Design review of the part built by this model. Coordinates are the model's own, in mm. Face numbers are marked on the shaded views. A direction names the side the tool comes from. Coordinates: 2 decimals unless noted, no trailing zeros. Loops run counter-clockwise (first coordinate to the right, second up) from the corner with the lowest first, then second, coordinate; pieces in that order, holes last. Notation, with made-up numbers: (-13.75, 22) -> (33.25, 22) arc R26 cw to (33.25, 36) -> close; hole circle Ø8 at (7.25, 0.5). An arc over 180 degrees is marked (long way). Answer as a JSON object with one key per item and string values.
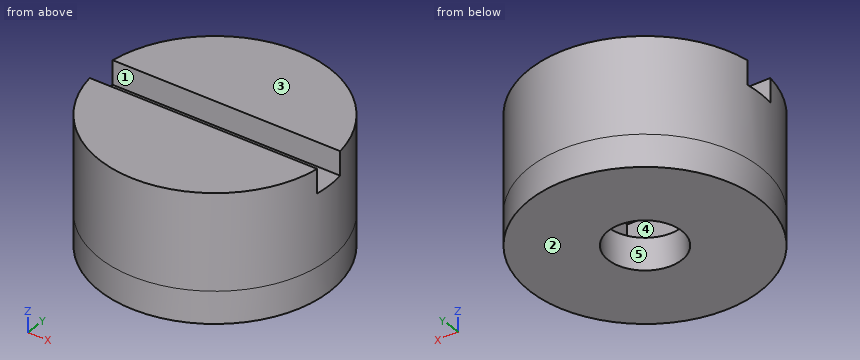
```python
from build123d import *

# Parameters (mm, degrees)
SKETCH_R        = 7.2
SKETCH_R_2      = 2.3
PAD_DEPTH       = 2
SKETCH001_R     = 7.2
PAD001_DEPTH    = 6
SKETCH002_W     = 8
SKETCH002_H     = 8
POCKET_DEPTH    = 3
SKETCH003_W     = 26.953154
SKETCH003_H     = 2
POCKET001_DEPTH = 3.5


with BuildPart() as part:
    # Sketch → Pad (new body)
    with BuildSketch(Plane.XY):
        Circle(SKETCH_R)
        Circle(SKETCH_R_2, mode=Mode.SUBTRACT)
    extrude(amount=-PAD_DEPTH)

    # Sketch001 → Pad001 (join)
    with BuildSketch(Plane.XY):
        Circle(SKETCH001_R)
    extrude(amount=PAD001_DEPTH)

    # Sketch002 → Pocket (cut)
    with BuildSketch(Plane.XY):
        Rectangle(SKETCH002_W, SKETCH002_H)
    extrude(amount=POCKET_DEPTH, mode=Mode.SUBTRACT)

    # Sketch003 (on DatumPlane) → Pocket001 (cut, symmetric)
    with BuildSketch(Plane.XY.offset(8)):
        Rectangle(SKETCH003_W, SKETCH003_H)
    extrude(amount=POCKET001_DEPTH, both=True, mode=Mode.SUBTRACT)


solid = part.part
```
1) Add section A-A, the plane y = 0. Give the boundary of the cut face in (x, z).
Completed:
{"outline": "(-7.2, -2) -> (-2.3, -2) -> (-2.3, 0) -> (-4, 0) -> (-4, 3) -> (4, 3) -> (4, 0) -> (2.3, 0) -> (2.3, -2) -> (7.2, -2) -> (7.2, 4.5) -> (-7.2, 4.5) -> close"}
2) Add section B-B, the plane x = 0. Give the boundary of the cut face in (y, z).
Completed:
{"outline": "(-7.2, -2) -> (-2.3, -2) -> (-2.3, 0) -> (-4, 0) -> (-4, 3) -> (4, 3) -> (4, 0) -> (2.3, 0) -> (2.3, -2) -> (7.2, -2) -> (7.2, 6) -> (1, 6) -> (1, 4.5) -> (-1, 4.5) -> (-1, 6) -> (-7.2, 6) -> close"}
3) Wall thickness on probe 1 along Z at (x, y) = (1.25, 2.5); probe 2 along X at (y, z) = (0.25, 2.75); probe 3 along Y at (x, z) = (0, -1.5): over which ranges is each line inside the solid? List them lowest first.
Completed:
{"probe 1": "-2 to 0, 3 to 6", "probe 2": "-7.2 to -4, 4 to 7.2", "probe 3": "-7.2 to -2.3, 2.3 to 7.2"}
4) Add section C-C, the plane z = 1.5. Give the boundary of the cut face in (x, y), and give its area (3 significant figures).
Completed:
{"outline": "circle Ø14.4 at (0, 0); hole (-4, -4) -> (4, -4) -> (4, 4) -> (-4, 4) -> close", "area": "98.9 mm²"}
5) Clearance check with flat-ended pins moving along their axes: pin 1 Ø1 at (y, z) = (4.5, 3) entering from -X; pin 2 Ø1.5 at (y, z) = (-1, 1) entering from -X; pin 3 Ø3 at (x, z) = (-4, 3.5) entering from -Y. State where each tip first meets the part, or that it passes through.
Completed:
{"pin 1": "x = -5.99", "pin 2": "x = -7.2", "pin 3": "y = -6.75"}
6) For the marked faces 1 and 2, list the 3-axis set-ups (+Z, -Z, +X, -X, +Y, -Y) from which the entire face can be reached by the end or side of a thin tool; tool diameter is ignored.
Completed:
{"face 1": "+Z, +X, -X", "face 2": "-Z, +X, -X, +Y, -Y"}
7) The part is to be moulded in two halves that separate along Z. For the marked faces 3, 4 and 5, say which applies: pulls with the +Z half, pulls with the -Z half, needs draft (parallel to the pull), parting line crosses it, or undercut.
Completed:
{"face 3": "pulls with the +Z half", "face 4": "undercut", "face 5": "needs draft"}
8) Add section D-D, the plane z = 5.5. Give the boundary of the cut face in (x, y).
Completed:
{"outline": "(-7.13, -1) arc R7.2 ccw to (7.13, -1) -> close; (-7.13, 1) -> (7.13, 1) arc R7.2 ccw to start"}
